```python
from build123d import *

# Parameters (mm, degrees)
F1_DEPTH = 0.6
F3_DEPTH = 4
F4_SIZE  = 1
F5_SIZE2 = 1.5
F5_SIZE  = 3
F6_R     = 2
F7_W     = 5
F7_H     = 0.6
F8_DEPTH = 25
F9_SIZE  = 0.4


with BuildPart() as f1:
    # F0 (on Top) → F1 (new body)
    with BuildSketch(Plane.XY):
        with BuildLine():
            ThreePointArc((0, 5), (1.4644660941, 1.4644660941), (5, 0))
            Line((5, 0), (8, 0))
            Line((8, 0), (8, 8.5))
            Line((8, 8.5), (33, 8.5))
            Line((33, 8.5), (33, 0))
            Line((33, 0), (36, 0))
            ThreePointArc((36, 0), (39.5355339059, 1.4644660941), (41, 5))
            Line((41, 5), (41, 12))
            ThreePointArc((41, 12), (39.5355339059, 15.5355339059), (36, 17))
            Line((36, 17), (5, 17))
            ThreePointArc((5, 17), (1.4644660941, 15.5355339059), (0, 12))
            Line((0, 12), (0, 5))
        make_face()
    extrude(amount=F1_DEPTH)

    # F2 (on face) → F3 (join)
    with BuildSketch(Plane.XY.offset(0.6)):
        Polygon((36, 12), (5, 12), (5, 5), (8, 5), (8, 8.5), (33, 8.5), (33, 5), (36, 5), align=None)
    extrude(amount=F3_DEPTH)

    # F4
    f4_edges = [f1.edges().sort_by_distance(p)[0] for p in [
        (5, 8.5, 4.6),
        (20.5, 12, 4.6),
        (36, 8.5, 4.6),
    ]]
    chamfer(f4_edges, length=F4_SIZE)

    # F5
    f5_edges = [f1.edges().sort_by_distance(p)[0] for p in [
        (20.5, 8.5, 0),
    ]]
    f5_side = f1.faces().sort_by_distance((20.5, 8.5, 2.3))[0]
    chamfer(f5_edges, length=F5_SIZE, length2=F5_SIZE2, reference=f5_side)

    # F6
    f6_edges = [f1.edges().sort_by_distance(p)[0] for p in [
        (20.5, 10, 0),
        (20.5, 8.5, 3),
    ]]
    fillet(f6_edges, radius=F6_R)

    # F7 (on face) → F8 (join, through all)
    with BuildSketch(Plane.YZ.offset(8)):
        with Locations((2.5, 0.3)):
            Rectangle(F7_W, F7_H)
    extrude(amount=F8_DEPTH)

    # F9
    f9_edges = [f1.edges().sort_by_distance(p)[0] for p in [
        (20.5, 17, 0),
        (20.5, 5, 0),
        (8, 8.118034, 0),
        (41, 8.5, 0),
        (39.535534, 1.464466, 0),
        (20.5, 0, 0),
        (1.464466, 1.464466, 0),
        (0, 8.5, 0),
        (1.464466, 15.535534, 0),
        (39.535534, 15.535534, 0),
        (33, 8.118034, 0),
    ]]
    chamfer(f9_edges, length=F9_SIZE)


solid = f1.part
```
Source: CAD feature listing. Evaluate the final solid. Frame: model axes, mm. A direction names the side the tool comes from. Give positions to 0.01 mm unless a question says otherwise; leave off trailing zeros. Write each loop counter-clockwise with the first axis right and the second up, starting at its lowest first coordinate (ties: lowest second). Pieces come first, ordered by that corner, then holes.
1. Material intervals for line 1 along X through (y, z) = (5.25, 1.3); line 2 along X through (y, z) = (10.75, 2.1); line 3 along Z through (x, y) = (23, 16), sorted ascending.
2. Section query C-C (z = 4). Return the cut outline in (x, y), then the cut area to 3 significant figures.
3. First-contact query: pin 1 (0.6 mm diameter, centred on x = 26.5, z = 4.5, fed in from -Y); pin 2 (2.5 mm diameter, centred on x = 7, z = 2, fed in from -Y); pin 3 (0.9 mm diameter, centred on x = 13, z = 2, fed in from +Y). Flat tips, straight axial feed; report the tip coordinate or a pass-through.
4. Section query D-D (z = 1.8). Return the cut outline in (x, y), then the cut area to 4 significant figures.
5. Section query B-B (y = 6). Return the cut outline in (x, z).
6. Pull-direction query (X, two-part tool) for faces 5 (the face through (36, 8, 2)), 6 (the face through (8, 7, 2)), 7 (the face through (5, 9, 2)), 8 (the face through (20.68, 10.17, 0.31)); classes: +X half, -X half, draft (parallel to the pull), parting line (faces both ways), or undercut.
7. Section query A-A (x = 16.5). Return the cut outline in (y, z), then the cut area to 3 significant figures.
8. Access query for faces 1 (the face through (20, 9, 2)), 2 (the face through (21, 12, 2)), 3 (the face through (34, 5, 3)), 4 (the face through (1.704, 15.37, 0.114)). Directions: +Z, -Z, +X, -X, +Y, -Y. A direction counts if a zero-diameter tool reaches every point of the face in a straight line with its end or side. Return the directions, or none.
Output values:
1. line 1: x = 5 to 8, 33 to 36
1. line 2: x = 5 to 36
1. line 3: z = 0 to 0.6
2. outline: (5.4, 5) - (8, 5) - (8, 8.5) - (33, 8.5) - (33, 5) - (35.6, 5) - (35.6, 11.6) - (5.4, 11.6) - close
2. area: 112 mm2
3. pin 1: stops at y = 8.5
3. pin 2: stops at y = 5
3. pin 3: stops at y = 12
4. outline: (5, 5) - (8, 5) - (8, 9.1) - (33, 9.1) - (33, 5) - (36, 5) - (36, 12) - (5, 12) - close
4. area: 114.5 mm2
5. outline: (0, 0.4) - (0.4, 0) - (7.6, 0) - (8, 0.4) - (8, 4.6) - (6, 4.6) - (5, 3.6) - (5, 0.6) - (0, 0.6) - close; (33, 0.4) - (33.4, 0) - (40.6, 0) - (41, 0.4) - (41, 0.6) - (36, 0.6) - (36, 3.6) - (35, 4.6) - (33, 4.6) - close
6. face 5: +X half
6. face 6: undercut
6. face 7: -X half
6. face 8: undercut
7. outline: (0, 0.4) - (0.4, 0) - (4.6, 0) - (5, 0.4) - (5, 0.6) - (0, 0.6) - close; (8.5, 3.47) arc R2 ccw to (8.71, 2.58) - (9.45, 1.11) arc R2 ccw to (11.24, 0) - (16.6, 0) - (17, 0.4) - (17, 0.6) - (12, 0.6) - (12, 3.6) - (11, 4.6) - (8.5, 4.6) - close
7. area: 18.8 mm2
8. face 1: -Z, -Y
8. face 2: +Z, +X, -X, +Y
8. face 3: +Z, +X, -X, -Y
8. face 4: -Z, -X, +Y
